Geometry: final body of the model. Coordinates: model frame, mm. Face numbers are marked on the shaded views. Give positions to 0.01 mm unless a question says otherwise; leave off trailing zeros. Loops run counter-clockwise (first coordinate to the right, second up) from the corner with the lowest first, then second, coordinate; pieces in that order, holes last. Notation, with made-up numbers: (33.25, 3) - (49.25, 3) arc R29 ccw to (49.25, 42) - close; hole circle Ø8 at (-34, 12.25). An arc over 180 degrees is marked (long way). Use one line per item in the form item = value.
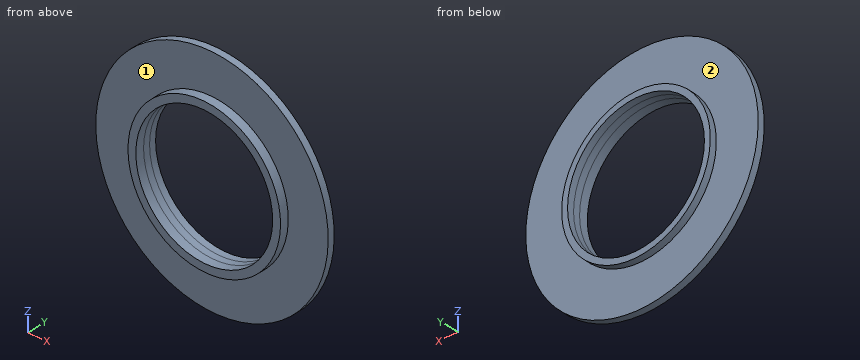
```python
from build123d import *
from build123d.topology import SkipClean

# Parameters (mm, degrees)
CROQUIS1_R              = 35.597110005
CROQUIS1_R_2            = 26.191176114
SALIENTE_EXTRUIR1_DEPTH = 1.5
CROQUIS2_R              = 60.448384053
SALIENTE_EXTRUIR2_DEPTH = 3.5
CROQUIS3_R              = 38.685318644
CROQUIS3_R_2            = 35.604684405
SALIENTE_EXTRUIR3_DEPTH = 3.5
CROQUIS4_R              = 35.604684405
CORTAR_EXTRUIR1_DEPTH   = 86.558542935
CROQUIS5_R              = 39.680725698
CROQUIS5_R_2            = 35.604684405
SALIENTE_EXTRUIR4_DEPTH = 4.5


with BuildPart() as part:
    # Croquis1 → Saliente-Extruir1 (new body)
    with BuildSketch(Plane(origin=(0, 0, 0), x_dir=(1, 0, 0), z_dir=(0, 1, 0))):
        with Locations(Location((0, 0, 0), (0, 0, 270))):
            Circle(CROQUIS1_R)
        with Locations(Location((0, 0, 0), (0, 0, 270))):
            Circle(CROQUIS1_R_2, mode=Mode.SUBTRACT)
    extrude(amount=SALIENTE_EXTRUIR1_DEPTH)

    # Croquis2 → Saliente-Extruir2 (add)
    with BuildSketch(Plane(origin=(0, 1.5, 0), x_dir=(1, 0, 0), z_dir=(0, 1, 0))):
        with Locations(Location((0, 0, 0), (0, 0, 270))):
            Circle(CROQUIS2_R)
    extrude(amount=-SALIENTE_EXTRUIR2_DEPTH)

    # Croquis3 → Saliente-Extruir3 (add)
    with BuildSketch(Plane(origin=(0, 1.5, 0), x_dir=(1, 0, 0), z_dir=(0, 1, 0))):
        with Locations(Location((0, 0, 0), (0, 0, 270))):
            Circle(CROQUIS3_R)
        with Locations(Location((0, 0, 0), (0, 0, 270))):
            Circle(CROQUIS3_R_2, mode=Mode.SUBTRACT)
    extrude(amount=SALIENTE_EXTRUIR3_DEPTH)

    # Croquis4 → Cortar-Extruir1 (cut, through all)
    with BuildSketch(Plane(origin=(0, 1.5, 0), x_dir=(1, 0, 0), z_dir=(0, 1, 0))):
        with Locations(Location((0, 0, 0), (0, 0, 270))):
            Circle(CROQUIS4_R)
    extrude(amount=-CORTAR_EXTRUIR1_DEPTH, mode=Mode.SUBTRACT)

    # Croquis5 → Saliente-Extruir4 (add)
    with SkipClean():  # the faces are left unmerged after this step: merging them gives an invalid solid
        with BuildSketch(Plane(origin=(0, -2, 0), x_dir=(-1, 0, 0), z_dir=(0, -1, 0))):
            with Locations(Location((0, 0, 0), (0, 0, 270))):
                Circle(CROQUIS5_R)
            with Locations(Location((0, 0, 0), (0, 0, 90))):
                Circle(CROQUIS5_R_2, mode=Mode.SUBTRACT)
        extrude(amount=SALIENTE_EXTRUIR4_DEPTH)
    add(part.part.scale(1), mode=Mode.REPLACE)  # the faces are merged on a copy


solid = part.part
```
(1) Pull-direction query (Y, two-part tool) for the marked faces 1 and 2; classes: released by +Y, released by -Y, zero draft, split by the parting line, or undercut.
Solution:
face_1 = released by -Y
face_2 = released by +Y
(2) Cut plane C-C (y = -5). Return the cut outline in (x, z), plus the area to 3 significant figures.
Solution:
outline = circle Ø79.36 at (0, 0); hole circle Ø71.21 at (0, 0)
area = 964 mm2
(3) Cut plane A-A (z = 0). Return the cut outline in (x, y), plus the area to 3 significant figures.
Solution:
outline = (-60.45, -2) - (-39.68, -2) - (-39.68, -6.5) - (-35.6, -6.5) - (-35.6, 5) - (-38.69, 5) - (-38.69, 1.5) - (-60.45, 1.5) - close; (35.6, -6.5) - (39.68, -6.5) - (39.68, -2) - (60.45, -2) - (60.45, 1.5) - (38.69, 1.5) - (38.69, 5) - (35.6, 5) - close
area = 232 mm2
(4) Cut plane D-D (z = 52.5). Return the cut outline in (x, y), plus the area to 3 significant figures.
Solution:
outline = (-29.96, -2) - (29.96, -2) - (29.96, 1.5) - (-29.96, 1.5) - close
area = 210 mm2
(5) Material intervals for L1, parallel to X at y = -0.75, z = 0; L2, parallel to X at y = -5, z = 0; L3, parallel to Y at x = -46, z = 10.5, sorted ascending. Write a range as from..to.
Solution:
L1 = -60.45..-35.6, 35.6..60.45
L2 = -39.68..-35.6, 35.6..39.68
L3 = -2..1.5
(6) Pin query (flat end, axial travel): P1, Ø1.5, axis at y = -0.5, z = -20, coming from the -X side; P2, Ø1.5, axis at y = -1.5, z = 40, coming from the +X side; P3, Ø3, axis at x = 19.5, y = -0.5, coming from the +Z side. Return the tip coordinate at first contact, or that it passes through.
Solution:
P1 = -57.3
P2 = 45.97
P3 = 57.71
(7) Cut plane B-B (x = 0). Return the cut outline in (y, z).
Solution:
outline = (-6.5, -39.68) - (-2, -39.68) - (-2, -60.45) - (1.5, -60.45) - (1.5, -38.69) - (5, -38.69) - (5, -35.6) - (-6.5, -35.6) - close; (-6.5, 35.6) - (5, 35.6) - (5, 38.69) - (1.5, 38.69) - (1.5, 60.45) - (-2, 60.45) - (-2, 39.68) - (-6.5, 39.68) - close
